Check sheet for the drawn part. Datum: minimum x, y, z corner. Units: mm. A direction names the side the tool comes from. Round coordinates to 2 decimals unless told otherwise and drop trailing zeros. Write each loop counter-clockwise with the first axis right and the second up, starting at its lowest first coordinate (ties: lowest second). Pieces come first, ordered by that corner, then holes. Notation, with made-up numbers: (-1, 65) -> (52, 65) arc R24 cw to (52, 82) -> close; hole circle Ø9 at (-28, 69.5). An arc over 180 degrees is marked (long way). One line per item, written item: value.
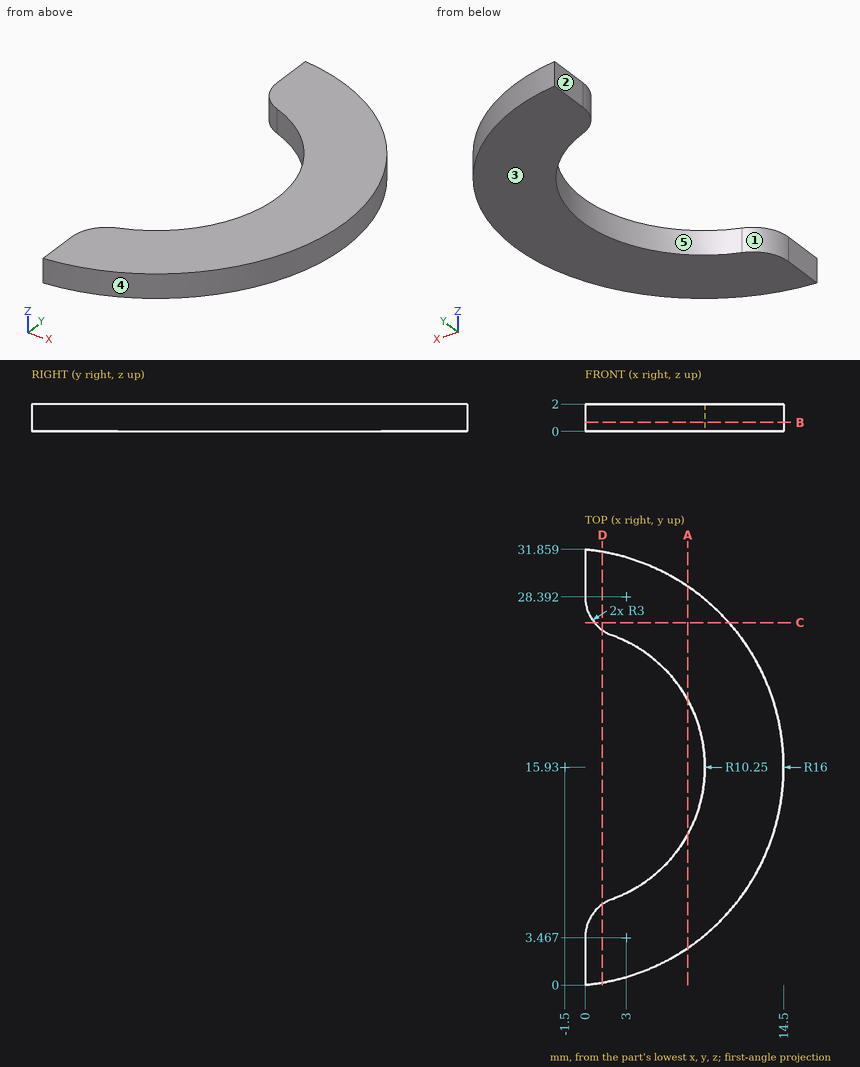
Item 1: Mould release check, pull along Y, two halves, no side actions. Record for the marked faces 3, 4 and 5: pulls with the +Y half, pulls with the -Y half, needs draft (parallel to the pull), parting line crosses it, or undercut.
Answer:
face 3: needs draft
face 4: parting line crosses it
face 5: undercut
Item 2: Sectioned sample at C-C on y = 26.5. Enter the section's corners in (x, z).
Answer:
outline: (0.67, 0) -> (10.51, 0) -> (10.51, 2) -> (0.67, 2) -> close
Item 3: Sectioned sample at D-D on x = 1.25. Enter the section's corners in (y, z) (1 decimal).
Answer:
outline: (0.2, 0) -> (5.9, 0) -> (5.9, 2) -> (0.2, 2) -> close; (26, 0) -> (31.7, 0) -> (31.7, 2) -> (26, 2) -> close
Item 4: Sectioned sample at A-A on x = 7.5. Enter the section's corners in (y, z) (1 decimal), and give its area (3 significant figures).
Answer:
outline: (2.7, 0) -> (11, 0) -> (11, 2) -> (2.7, 2) -> close; (20.8, 0) -> (29.2, 0) -> (29.2, 2) -> (20.8, 2) -> close
area: 33.3 mm^2
Item 5: Depth check by flat-ended pin: P1, Ø1, axis at y = 10, z = 1.5, coming from the +X side; P2, Ø1, axis at x = 6.5, z = 1.5, coming from the -Y side (1 decimal). Enter the tip coordinate at first touch or a pass-through.
Answer:
P1: stops at x = 13.55
P2: stops at y = 1.8
Item 6: Tool access check on the marked faces 1 and 2. Record the directions out of +Z, -Z, +X, -X, +Y, -Y that give a thin tool (end or side, any length) a straight path to the whole face; none if there is none.
Answer:
face 1: +Z, -Z, -X
face 2: +Z, -Z, -X, +Y, -Y
Item 7: Sectioned sample at B-B on z = 0.65. Enter the section's corners in (x, y), and give its area (3 significant figures).
Answer:
outline: (0, 0) arc R16 ccw to (0, 31.86) -> (0, 28.39) arc R3 ccw to (1.98, 25.57) arc R10.25 cw to (1.98, 6.29) arc R3 ccw to (0, 3.47) -> close
area: 218 mm^2
Item 8: Thickness scan on line 1 (Y direction, x = 6, z = 1.95) (1 decimal); line 2 (Y direction, x = 1.75, z = 0.4) (1 decimal); line 3 (Y direction, x = 9.5, z = 0.95). Record the ranges inside material, lowest first.
Answer:
line 1: y = 1.8 to 8.9, 22.9 to 30.1
line 2: y = 0.3 to 6.2, 25.7 to 31.6
line 3: y = 4.31 to 27.55
